from build123d import *

# Parameters (mm, degrees)
SKETCH_1_W                       = 4
SKETCH_1_H                       = 4
EXTRUDE_1_DEPTH                  = 100
FILLET_1_R                       = 1
FILLET_2_R                       = 2
FILLET_3_R                       = 0.5
PATTERN_CIRCULAR_1_COUNT         = 4
FILLET_1_OF_PATTERN_CIRCULAR_1_R = 1
FILLET_2_OF_PATTERN_CIRCULAR_1_R = 2
FILLET_3_OF_PATTERN_CIRCULAR_1_R = 0.5
SKETCH_2_R                       = 3.4
CUT_EXTRUDE_1_DEPTH              = 101
SKETCH_3_R                       = 4
CUT_EXTRUDE_2_DEPTH              = 15


with BuildPart() as part:
    # 草图1 → 凸台-拉伸1 (new body)
    with BuildSketch(Plane.XY):
        Polygon((5.7, 0), (5.7, 4.427207794), (9.672792206, 8.4), (13.2, 8.4), (13.2, 4.1), (14.1, 4.1), (14.1, 5.1), (15, 5.1), (15, 15), (5.1, 15), (5.1, 14.1), (4.1, 14.1), (4.1, 13.2), (8.4, 13.2), (8.4, 9.672792206), (4.427207794, 5.7), (0, 5.7), (0, 0), align=None)
        with Locations((11.7, 11.7)):
            Rectangle(SKETCH_1_W, SKETCH_1_H, mode=Mode.SUBTRACT)
    extrude_1 = extrude(amount=EXTRUDE_1_DEPTH)

    # 圆角1
    fillet_1_edges = [part.edges().sort_by_distance(p)[0] for p in [
        (13.7, 9.7, 50),
        (13.7, 13.7, 50),
        (9.7, 13.7, 50),
        (9.7, 9.7, 50),
    ]]
    fillet(fillet_1_edges, radius=FILLET_1_R)

    # 圆角2
    fillet_2_edges = [part.edges().sort_by_distance(p)[0] for p in [
        (15, 15, 50),
    ]]
    fillet(fillet_2_edges, radius=FILLET_2_R)

    # 圆角3
    fillet_3_edges = [part.edges().sort_by_distance(p)[0] for p in [
        (4.427207794, 5.7, 50),
        (8.4, 9.672792206, 50),
        (8.4, 13.2, 50),
        (13.2, 8.4, 50),
        (9.672792206, 8.4, 50),
        (5.7, 4.427207794, 50),
    ]]
    fillet(fillet_3_edges, radius=FILLET_3_R)

    # 阵列(圆周)1: 凸台-拉伸1 ×4 about axis
    pattern_circular_1_axis = Axis((0, 0, 0), (0, 0, 1))
    for i in range(1, PATTERN_CIRCULAR_1_COUNT):
        add(extrude_1.rotate(pattern_circular_1_axis, i * 360 / PATTERN_CIRCULAR_1_COUNT))

    # 圆角1 of 阵列(圆周)1
    fillet_1_of_pattern_circular_1_edges = [part.edges().sort_by_distance(p)[0] for p in [
        (-9.7, 13.7, 50),
        (-13.7, 13.7, 50),
        (-13.7, 9.7, 50),
        (-9.7, 9.7, 50),
        (-13.7, -9.7, 50),
        (-13.7, -13.7, 50),
        (-9.7, -13.7, 50),
        (-9.7, -9.7, 50),
        (9.7, -13.7, 50),
        (13.7, -13.7, 50),
        (13.7, -9.7, 50),
        (9.7, -9.7, 50),
    ]]
    fillet(fillet_1_of_pattern_circular_1_edges, radius=FILLET_1_OF_PATTERN_CIRCULAR_1_R)

    # 圆角2 of 阵列(圆周)1
    fillet_2_of_pattern_circular_1_edges = [part.edges().sort_by_distance(p)[0] for p in [
        (-15, 15, 50),
        (-15, -15, 50),
        (15, -15, 50),
    ]]
    fillet(fillet_2_of_pattern_circular_1_edges, radius=FILLET_2_OF_PATTERN_CIRCULAR_1_R)

    # 圆角3 of 阵列(圆周)1
    fillet_3_of_pattern_circular_1_edges = [part.edges().sort_by_distance(p)[0] for p in [
        (-5.7, 4.427207794, 50),
        (-9.672792206, 8.4, 50),
        (-13.2, 8.4, 50),
        (-8.4, 13.2, 50),
        (-8.4, 9.672792206, 50),
        (-4.427207794, 5.7, 50),
        (-4.427207794, -5.7, 50),
        (-8.4, -9.672792206, 50),
        (-8.4, -13.2, 50),
        (-13.2, -8.4, 50),
        (-9.672792206, -8.4, 50),
        (-5.7, -4.427207794, 50),
        (5.7, -4.427207794, 50),
        (9.672792206, -8.4, 50),
        (13.2, -8.4, 50),
        (8.4, -13.2, 50),
        (8.4, -9.672792206, 50),
        (4.427207794, -5.7, 50),
    ]]
    fillet(fillet_3_of_pattern_circular_1_edges, radius=FILLET_3_OF_PATTERN_CIRCULAR_1_R)

    # 草图2 → 切除-拉伸1 (cut, through all)
    with BuildSketch(Plane.XY.offset(100)):
        Circle(SKETCH_2_R)
    extrude(amount=-CUT_EXTRUDE_1_DEPTH, mode=Mode.SUBTRACT)

    # 草图3 → 切除-拉伸2 (cut, symmetric)
    with BuildSketch(Plane(origin=(0, 0, 0), x_dir=(0, 0, -1), z_dir=(1, 0, 0))):
        with Locations((-80.8, 0)):
            Circle(SKETCH_3_R)
    extrude(amount=CUT_EXTRUDE_2_DEPTH, both=True, mode=Mode.SUBTRACT)


solid = part.part
Geometry check sheet. Reference: the model listing, model coordinates, mm. A direction names the side the tool comes from. Round coordinates to 2 decimals unless told otherwise and drop trailing zeros. Loops run counter-clockwise (first coordinate to the right, second up) from the corner with the lowest first, then second, coordinate; pieces in that order, holes last. Notation, with made-up numbers: (-7.75, 33) -> (36.25, 33) arc R26 ccw to (36.25, 67) -> close; hole circle Ø3 at (-26.5, 8). An arc over 180 degrees is marked (long way). Answer as a JSON object with one key per item and string values. Group by question number.
Item 1: Cross-section at B-B, the plane x = 0. Record the cut outline in (y, z).
Item 2: Depth check by flat-ended pin: pin 1 Ø6.5 at (y, z) = (0, 80.8) entering from -X; pin 2 Ø0.8 at (x, z) = (-4.5, 41.5) entering from +Y; pin 3 Ø1 at (x, z) = (-14.5, 42.5) entering from +Y; pin 4 Ø0.7 at (y, z) = (14.5, 64) entering from -X. Enter the tip coordinate at first touch or a pass-through.
Item 3: Release check for a two-part mould opening along Y. For faces 1 (the face through (12, -13.7, 49)), 2 (the face through (-9, -15, 49)), 3 (the face through (9.7, -12, 49)), 4 (the face through (9, 15, 49)) record: pulls with the +Y half, pulls with the -Y half, needs draft (parallel to the pull), parting line crosses it, or undercut.
Item 4: Cross-section at A-A, the plane y = 0. Record the cut outline in (x, z).
Item 5: Thickness scan on line 1 along Y through (x, z) = (10.5, 42.5); line 2 along X through (y, z) = (-11, 5.5); line 3 along X through (y, z) = (0, 89.25). Record the ranges inside material, lowest first.
Item 6: Cross-section at C-C, the plane z = 80.8. Count the separate pieces of the cut face and the enclosed holes in it, plus the area to 3 significant figures.
Item 7: Set-up check for faces 5 (the face through (6, 13.2, 49)), 6 (the face through (-14.4, 14.43, 50.7)): record each of +Z, -Z, +X, -X, +Y, -Y from which the full face is reachable in a straight line by a thin tool's end or side.
Determined:
{
 "1": {"outline": "(-5.7, 0) -> (-3.4, 0) -> (-3.4, 78.69) arc R4 cw to (-3.4, 82.91) -> (-3.4, 100) -> (-5.7, 100) -> close; (3.4, 0) -> (5.7, 0) -> (5.7, 100) -> (3.4, 100) -> (3.4, 82.91) arc R4 cw to (3.4, 78.69) -> close"},
 "2": {"pin 1": "passes through", "pin 2": "stops at y = 14.1", "pin 3": "stops at y = 14.73", "pin 4": "stops at x = -14.64"},
 "3": {"face 1": "undercut", "face 2": "pulls with the -Y half", "face 3": "undercut", "face 4": "pulls with the +Y half"},
 "4": {"outline": "(-5.7, 0) -> (-3.4, 0) -> (-3.4, 76.8) -> (-5.7, 76.8) -> close; (-5.7, 84.8) -> (-3.4, 84.8) -> (-3.4, 100) -> (-5.7, 100) -> close; (3.4, 0) -> (5.7, 0) -> (5.7, 76.8) -> (3.4, 76.8) -> close; (3.4, 84.8) -> (5.7, 84.8) -> (5.7, 100) -> (3.4, 100) -> close"},
 "5": {"line 1": "y = -15 to -13.68, -9.72 to -8.4, 8.4 to 9.72, 13.68 to 15", "line 2": "x = -15 to -13.7, -9.7 to -8.4, 8.4 to 9.7, 13.7 to 15", "line 3": "x = -5.7 to -3.4, 3.4 to 5.7"},
 "6": {"separate pieces": "2", "enclosed holes": "4", "area": "238 mm²"},
 "7": {"face 5": "+Z, -Z", "face 6": "+Z, -Z, -X, +Y"}
}
